from build123d import *

# Parameters (mm, degrees)
SKETCH1_W           = 194
SKETCH1_H           = 152
BOSS_EXTRUDE1_DEPTH = 104
SHELL1_T            = -1.5
CUT_EXTRUDE1_DEPTH  = 2
SKETCH4_W           = 104
SKETCH4_H           = 8.8
BOSS_EXTRUDE2_DEPTH = 9.5
FILLET1_R           = 10
FILLET2_R           = 2


with BuildPart() as part:
    # Sketch1 → Boss-Extrude1 (new body)
    with BuildSketch(Plane.YZ):
        with Locations((97, -76)):
            Rectangle(SKETCH1_W, SKETCH1_H)
    extrude(amount=BOSS_EXTRUDE1_DEPTH)

    # Shell1
    shell1_openings = [part.faces().sort_by_distance(p)[0] for p in [
        (52, 97, -152),
    ]]
    offset(amount=SHELL1_T, openings=shell1_openings, kind=Kind.INTERSECTION)

    # Sketch2 → Cut-Extrude1 (cut)
    with BuildSketch(Plane(origin=(0, 0, 0), x_dir=(0, -1, 0), z_dir=(-1, 0, 0))):
        Polygon((-192.5, -1.5), (-192.5, -150.5), (-192.5, -152), (-1.5, -152), (-1.5, -150.5), (-1.5, -1.5), align=None)
    extrude(amount=-CUT_EXTRUDE1_DEPTH, mode=Mode.SUBTRACT)

    # Sketch4 → Boss-Extrude2 (add)
    with BuildSketch(Plane(origin=(0, 0, -152), x_dir=(1, 0, 0), z_dir=(0, 0, -1))):
        with Locations((52, 2.9)):
            Rectangle(SKETCH4_W, SKETCH4_H)
        with Locations((52, -196.9)):
            Rectangle(SKETCH4_W, SKETCH4_H)
    extrude(amount=BOSS_EXTRUDE2_DEPTH)

    # Fillet1
    # the kernel refuses this fillet: 10 mm, written as the material it adds along each edge
    with BuildSketch(Plane(origin=(0, 0, -152), x_dir=(0, -1, 0), z_dir=(1, 0, 0))) as fillet1_piece_1:
        with BuildLine():
            CenterArc((10, -9.628603222), FILLET1_R, 105.664266851, 74.335733149)
            Line((0, -9.628603222), (-0.2, -9.628603222))
            Line((-0.2, -9.628603222), (-0.2, 0))
            Line((-0.2, 0), (0, 0.2))
            ThreePointArc((0, 0.2), (3.65, 0.2), (7.246, 0.192572064))
            Line((7.246, 0.192572064), (7.3, 0))
        make_face()
    extrude(amount=104)
    with BuildSketch(Plane(origin=(0, 194, -152), x_dir=(0, 1, 0), z_dir=(1, 0, 0))) as fillet1_piece_2:
        with BuildLine():
            CenterArc((10, 9.628603222), FILLET1_R, 180, 74.335733149)
            Line((0, 9.628603222), (-0.2, 9.628603222))
            Line((-0.2, 9.628603222), (-0.2, 0))
            Line((-0.2, 0), (0, -0.2))
            ThreePointArc((0, -0.2), (3.65, -0.2), (7.246, -0.192572064))
            Line((7.246, -0.192572064), (7.3, 0))
        make_face()
    extrude(amount=104)

    # Fillet2
    # the kernel refuses this fillet: 2 mm, written as the material it takes off along each edge
    with BuildSketch(Plane(origin=(102, 2, -2), x_dir=(1, 0, 0), z_dir=(0, -1, 0))) as fillet2_piece_1_section:
        Polygon((0, 0), (FILLET2_R, 0), (FILLET2_R, FILLET2_R), (0, FILLET2_R), align=None)
    fillet2_piece_1 = extrude(amount=FILLET2_R, mode=Mode.PRIVATE)
    fillet2_piece_1 = fillet2_piece_1 - Plane(origin=(102, 2, -2), x_dir=(-0.7071067811865475, 0, -0.7071067811865475), z_dir=(0, -1, 0)) * Sphere(FILLET2_R, mode=Mode.PRIVATE)
    add(fillet2_piece_1, mode=Mode.SUBTRACT)
    with BuildSketch(Plane(origin=(102, 192, -2), x_dir=(1, 0, 0), z_dir=(0, 1, 0))) as fillet2_piece_2_section:
        Polygon((0, 0), (FILLET2_R, 0), (FILLET2_R, -FILLET2_R), (0, -FILLET2_R), align=None)
    fillet2_piece_2 = extrude(amount=FILLET2_R, mode=Mode.PRIVATE)
    fillet2_piece_2 = fillet2_piece_2 - Plane(origin=(102, 192, -2), x_dir=(-0.7071067811865475, 0, -0.7071067811865475), z_dir=(0, 1, 0)) * Sphere(FILLET2_R, mode=Mode.PRIVATE)
    add(fillet2_piece_2, mode=Mode.SUBTRACT)
    with BuildSketch(Plane(origin=(104, 2, 0), x_dir=(0, 0, -1), z_dir=(0, 1, 0))) as fillet2_piece_3:
        with BuildLine():
            CenterArc((FILLET2_R, FILLET2_R), FILLET2_R, 180, 90)
            Line((0, FILLET2_R), (0, 0))
            Line((0, 0), (FILLET2_R, 0))
        make_face()
    extrude(amount=190, mode=Mode.SUBTRACT)
    with BuildSketch(Plane(origin=(104, 0, -142.371396778), x_dir=(0, 1, 0), z_dir=(0, 0, 1))) as fillet2_piece_4:
        with BuildLine():
            CenterArc((FILLET2_R, FILLET2_R), FILLET2_R, 180, 90)
            Line((0, FILLET2_R), (0, 0))
            Line((0, 0), (FILLET2_R, 0))
        make_face()
    extrude(amount=140.371396778, mode=Mode.SUBTRACT)
    with BuildSketch(Plane(origin=(0, 0, -142.371396778), x_dir=(0, 1, 0), z_dir=(0, 0, 1))) as fillet2_piece_5:
        with BuildLine():
            CenterArc((FILLET2_R, -FILLET2_R), FILLET2_R, 90, 90)
            Line((0, -FILLET2_R), (0, 0))
            Line((0, 0), (FILLET2_R, 0))
        make_face()
    extrude(amount=147.371396778, mode=Mode.SUBTRACT)
    with BuildSketch(Plane(origin=(-5, 0, 0), x_dir=(0, 1, 0), z_dir=(1, 0, 0)), Plane(origin=(-5, 194, 0), x_dir=(0, 0, -1), z_dir=(1, 0, 0))) as fillet2_piece_6:
        with BuildLine():
            CenterArc((FILLET2_R, -FILLET2_R), FILLET2_R, 90, 90)
            Line((0, -FILLET2_R), (0, 0))
            Line((0, 0), (FILLET2_R, 0))
        make_face()
    extrude(amount=107, mode=Mode.SUBTRACT)
    with BuildSketch(Plane(origin=(0, 194, 5), x_dir=(1, 0, 0), z_dir=(0, 0, -1))) as fillet2_piece_7:
        with BuildLine():
            CenterArc((FILLET2_R, FILLET2_R), FILLET2_R, 180, 90)
            Line((0, FILLET2_R), (0, 0))
            Line((0, 0), (FILLET2_R, 0))
        make_face()
    extrude(amount=147.371396778, mode=Mode.SUBTRACT)
    with BuildSketch(Plane(origin=(104, 194, -2), x_dir=(-1, 0, 0), z_dir=(0, 0, -1))) as fillet2_piece_8:
        with BuildLine():
            CenterArc((FILLET2_R, -FILLET2_R), FILLET2_R, 90, 90)
            Line((0, -FILLET2_R), (0, 0))
            Line((0, 0), (FILLET2_R, 0))
        make_face()
    extrude(amount=140.371396778, mode=Mode.SUBTRACT)
    with BuildSketch(Plane(origin=(0, -10, -142.371396778), x_dir=(0, -0.2248060419259851, -0.9744035321742077), z_dir=(0, -0.9744035321742077, 0.2248060419259851))) as fillet2_piece_9:
        with BuildLine():
            CenterArc((10 + FILLET2_R, FILLET2_R), FILLET2_R, 180, 90)
            Line((10, FILLET2_R), (10, 0))
            Line((10, 0), (10 + FILLET2_R, 0))
        make_face()
    revolve(axis=Axis((0, -10, -142.371396778), (1, 0, 0)), revolution_arc=102.991472997, mode=Mode.SUBTRACT)
    with BuildSketch(Plane(origin=(104, -10, -142.371396778), x_dir=(0, -0.2248060419259851, -0.9744035321742077), z_dir=(0, -0.9744035321742077, 0.2248060419259851))) as fillet2_piece_10:
        with BuildLine():
            CenterArc((10 + FILLET2_R, -FILLET2_R), FILLET2_R, 90, 90)
            Line((10, -FILLET2_R), (10, 0))
            Line((10, 0), (10 + FILLET2_R, 0))
        make_face()
    revolve(axis=Axis((104, -10, -142.371396778), (1, 0, 0)), revolution_arc=102.991472997, mode=Mode.SUBTRACT)
    with BuildSketch(Plane(origin=(0, 204, -142.371396778), x_dir=(0, -1, 0), z_dir=(0, 0, 1))) as fillet2_piece_11:
        with BuildLine():
            CenterArc((10 + FILLET2_R, FILLET2_R), FILLET2_R, 180, 90)
            Line((10 + FILLET2_R, 0), (10, 0))
            Line((10, 0), (10, FILLET2_R))
        make_face()
    revolve(axis=Axis((0, 204, -142.371396778), (1, 0, 0)), revolution_arc=102.991472997, mode=Mode.SUBTRACT)
    with BuildSketch(Plane(origin=(104, 204, -142.371396778), x_dir=(0, -1, 0), z_dir=(0, 0, 1))) as fillet2_piece_12:
        with BuildLine():
            CenterArc((10 + FILLET2_R, -FILLET2_R), FILLET2_R, 90, 90)
            Line((10 + FILLET2_R, 0), (10, 0))
            Line((10, 0), (10, -FILLET2_R))
        make_face()
    revolve(axis=Axis((104, 204, -142.371396778), (1, 0, 0)), revolution_arc=102.991472997, mode=Mode.SUBTRACT)


solid = part.part
Check sheet for the modelled part. Datum: model origin and axes. Units: mm. A direction names the side the tool comes from. Round coordinates to 2 decimals unless told otherwise and drop trailing zeros. Loops run counter-clockwise (first coordinate to the right, second up) from the corner with the lowest first, then second, coordinate; pieces in that order, holes last. Notation, with made-up numbers: M 20,29 L 47,29 A24 cw 47,39 Z; hole C 30.5,3.25 d6. An arc over 180 degrees is marked long. One line per item, written item: value.
(1) Sectioned sample at C-C, the plane z = -68. Record the cut outline in (x, y).
Computed values:
outline: M 0.06,1.5 A2 ccw 2,0 L 102,0 A2 ccw 104,2 L 104,192 A2 ccw 102,194 L 2,194 A2 ccw 0.06,192.5 L 102.5,192.5 L 102.5,1.5 Z
(2) Access from +Z, -Z, +X, -X, +Y, -Y to the whole of each face (thin tool, end or side, straight path). Record for faces 5 (the face through (51, 194, -73)), 6 (the face through (102.5, 96, -76)), 7 (the face through (51, 197, -161.5)).
Computed values:
face 5: +Z, +X, -X, +Y
face 6: -Z, -X
face 7: -Z, +X, -X, +Y, -Y
(3) Release check for a two-part mould opening along Y. For faces 1 (the face through (51, 192.5, -83)), 2 (the face through (0, -2, -157)), 3 (the face through (51, 1.5, -80)), 4 (the face through (51, 0, -73)) record: +Y half, -Y half, draft (parallel to the pull), parting line (faces both ways), or undercut.
Computed values:
face 1: undercut
face 2: draft
face 3: undercut
face 4: -Y half
(4) Sectioned sample at A-A, the plane y = 12. Record the cut outline in (x, z).
Computed values:
outline: M 0,-1.5 L 102.5,-1.5 L 102.5,-152 L 104,-152 L 104,-2 A2 ccw 102,0 L 0,0 Z
(5) Sectioned sample at B-B, the plane x = 23.5. Record the cut outline in (y, z).
Computed values:
outline: M -7.3,-161.5 L 1.5,-161.5 L 1.5,-1.5 L 192.5,-1.5 L 192.5,-161.5 L 201.3,-161.5 L 201.3,-152 A10 cw 194,-142.37 L 194,-2 A2 ccw 192,0 L 2,0 A2 ccw 0,-2 L 0,-142.37 A10 cw -7.3,-152 Z
(6) Depth check by flat-ended pin: pin 1 Ø1 at (x, z) = (77.5, -96) entering from +Y; pin 2 Ø4 at (y, z) = (78.5, -51) entering from -X; pin 3 Ø1 at (x, y) = (62.5, 30.5) entering from +Z; pin 4 Ø8 at (x, y) = (56, 57.5) entering from -Z. Enter the tip coordinate at first touch or a pass-through.
Computed values:
pin 1: stops at y = 194
pin 2: stops at x = 102.5
pin 3: stops at z = 0
pin 4: stops at z = -1.5
(7) Thickness scan on line 1 (Y direction, x = 69, z = -103.5); line 2 (Z direction, x = 60.5, y = 2); line 3 (X direction, y = 122, z = -18). Record the ranges inside material, lowest first.
Computed values:
line 1: y = 0 to 1.5, 192.5 to 194
line 2: z = -1.5 to 0
line 3: x = 102.5 to 104
